Could you check a few things on this model? Use its own coordinates, in mm. Coordinates: 2 decimals unless noted, no trailing zeros. Order: outer loops, then holes, each group sorted by start corner. A loop starts at its lowest first (then second) coordinate and runs counter-clockwise, first axis right, second up. Notation, with made-up numbers: (-25.75, 27) -> (-8.75, 27) arc R28 ccw to (-8.75, 54) -> close; hole circle Ø10 at (52.25, 12.25). An arc over 180 degrees is marked (long way). Put each result on its own line as item: value. Start each with the question number.
Q1. Please list where this line runs through material, in increasing order: line 1 along X through (y, z) = (6, -269.5).
Q2. If we section it at A-A (y = 6): Please give me the cut outline in (x, z).
Q3. If we section it at B-B (z = -58): Please give me the cut outline in (x, y), and give its area (3 significant figures).
Q4. Will these pins go through, and if not, where does the flat tip stop? pin 1 (2 mm diameter, centred on y = 4.5, z = -252.5, fed in from +X); pin 2 (12 mm diameter, centred on x = 63.5, z = -264, fed in from -Y).
from build123d import *

# Parameters (mm, degrees)
SKETCH_1_W      = 200
SKETCH_1_H      = 450
EXTRUDE_1_DEPTH = 12
FILLET_1_R      = 10
SKETCH_2_R      = 3
EXTRUDE_2_DEPTH = 15


with BuildPart() as part:
    # 草图1 → 凸台-拉伸1 (new body)
    with BuildSketch(Plane(origin=(0, 0, 0), x_dir=(1, 0, 0), z_dir=(0, 1, 0))):
        with Locations((0, 225)):
            Rectangle(SKETCH_1_W, SKETCH_1_H)
    extrude(amount=EXTRUDE_1_DEPTH)

    # 圆角1
    fillet_1_edges = [part.edges().sort_by_distance(p)[0] for p in [
        (-100, 6, -450),
        (100, 6, -450),
        (100, 6, 0),
        (-100, 6, 0),
    ]]
    fillet(fillet_1_edges, radius=FILLET_1_R)

    # 草图2 → 凸台-拉伸2 (add)
    with BuildSketch(Plane(origin=(100, 0, 0), x_dir=(0, 0, -1), z_dir=(1, 0, 0))):
        with Locations(Location((225, 6, 0), (0, 0, 180))):
            Circle(SKETCH_2_R)
    extrude(amount=EXTRUDE_2_DEPTH)


solid = part.part
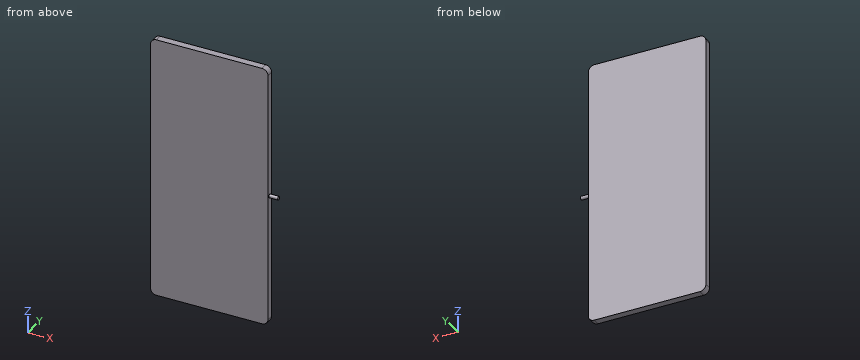
The answers:
1. line 1: -100 to 100
2. outline: (-100, -440) arc R10 ccw to (-90, -450) -> (90, -450) arc R10 ccw to (100, -440) -> (100, -228) -> (115, -228) -> (115, -222) -> (100, -222) -> (100, -10) arc R10 ccw to (90, 0) -> (-90, 0) arc R10 ccw to (-100, -10) -> close
3. outline: (-100, 0) -> (100, 0) -> (100, 12) -> (-100, 12) -> close
3. area: 2,400 mm^2
4. pin 1: x = 100
4. pin 2: y = 0
